from build123d import *

# Parameters (mm, degrees)
F0_W     = 120
F0_H     = 80
F1_DEPTH = 32
F2_W     = 40
F2_H     = 52
F3_DEPTH = 22
F4_W     = 40
F4_H     = 18
F5_DEPTH = 32.001
F6_W     = 30
F6_H     = 70
F7_DEPTH = 32.001
F9_DEPTH = 10


# Not quite as in the source:
# - a pattern or mirror of a feature is missing from the dataset's text; its kind, count and spacing are read off the source's solid


with BuildPart() as f1:
    # F0 (on Right) → F1 (new body)
    with BuildSketch(Plane.YZ):
        Rectangle(F0_W, F0_H)
    extrude(amount=-F1_DEPTH)

    # F2 (on face) → F3 (cut)
    with BuildSketch(Plane.YZ):
        with Locations((0, -14)):
            Rectangle(F2_W, F2_H)
    extrude(amount=-F3_DEPTH, mode=Mode.SUBTRACT)

    # F4 (on face) → F5 (cut, through all)
    with BuildSketch(Plane.YZ):
        with Locations((0, 31)):
            Rectangle(F4_W, F4_H)
    extrude(amount=-F5_DEPTH, mode=Mode.SUBTRACT)

    # F6 (on face) → F7 (cut, through all)
    with BuildSketch(Plane.YZ):
        with Locations((-45, 5)):
            Rectangle(F6_W, F6_H)
    f7 = extrude(amount=-F7_DEPTH, mode=Mode.SUBTRACT)

    # F7_copies: F7 across plane
    add(f7.mirror(Plane.ZX), mode=Mode.SUBTRACT)

    # F8 (on face) → F9 (join)
    with BuildSketch(Plane(origin=(-32, 0, 0), x_dir=(0, -1, 0), z_dir=(-1, 0, 0))):
        Polygon((60, -30), (30, 40), (30, -30), align=None)
    f9 = extrude(amount=-F9_DEPTH)

    # F9_copies: F9 across plane
    add(f9.mirror(Plane.ZX))


solid = f1.part
CAD build for the part. Positions are in the model's coordinates, mm. A direction names the side the tool comes from. Coordinates: 2 decimals unless noted, no trailing zeros. Order: outer loops, then holes, each group sorted by start corner. A loop starts at its lowest first (then second) coordinate and runs counter-clockwise, first axis right, second up.
Item 1: Band-saw the part on A-A on z = 25. List the corners of the cut face in (x, y).
Check sheet entries:
outline: (-32, -36.43) - (-22, -36.43) - (-22, -30) - (0, -30) - (0, -20) - (-32, -20) - close; (-32, 20) - (0, 20) - (0, 30) - (-22, 30) - (-22, 36.43) - (-32, 36.43) - close
Item 2: Pin check, flat tips, straight feed: pin 1 Ø9.5 at (x, y) = (-13.5, -5.5) entering from +Z; pin 2 Ø15 at (y, z) = (-41, 8.5) entering from +X; pin 3 Ø11 at (x, z) = (-8.5, -8.5) entering from -Y. Stop position of each tip, or through.
Check sheet entries:
pin 1: stops at z = 22
pin 2: stops at x = -22
pin 3: stops at y = -30
Item 3: Two-plate mould, pull along Y, no slides. Class faces 4 (the face through (-27, -45, 5)), 5 (the face through (-11, 0, 12)), 6 (the face through (-22, -38, -10)): +Y half, -Y half, draft (parallel to the pull), parting line (faces both ways), or undercut.
Check sheet entries:
face 4: -Y half
face 5: undercut
face 6: draft
Item 4: Band-saw the part on B-B on x = -14.5. List the corners of the cut face in (y, z), plus the area to 3 significant figures.
Check sheet entries:
outline: (-60, -40) - (-20, -40) - (-20, 12) - (20, 12) - (20, -40) - (60, -40) - (60, -30) - (30, -30) - (30, 40) - (20, 40) - (20, 22) - (-20, 22) - (-20, 40) - (-30, 40) - (-30, -30) - (-60, -30) - close
area: 2,600 mm2
Item 5: Band-saw the part on D-D on z = -22.5. List the corners of the cut face in (x, y), plus the area to 3 significant figures.
Check sheet entries:
outline: (-32, -56.79) - (-22, -56.79) - (-22, -30) - (0, -30) - (0, -20) - (-22, -20) - (-22, 20) - (0, 20) - (0, 30) - (-22, 30) - (-22, 56.79) - (-32, 56.79) - close
area: 1,580 mm2
Item 6: Band-saw the part on C-C on y = -48. List the corners of the cut face in (x, z), plus the area to 3 significant figures.
Check sheet entries:
outline: (-32, -40) - (0, -40) - (0, -30) - (-22, -30) - (-22, -2) - (-32, -2) - close
area: 600 mm2
Item 7: 3-axis set-ups, long thin cutter, end or side, ignore diameter. For faces 1 (the face through (-11, -20, -14)), 2 (the face through (-11, -30, 5)), 3 (the face through (-16, 20, 31)): which of +Z, -Z, +X, -X, +Y, -Y reach the whole face in a straight line?
Check sheet entries:
face 1: -Z, +X
face 2: +Z, +X, -Y
face 3: +Z, +X, -X
Item 8: Drill centre lines: L1, parallel to Y at x = -6, z = 23.5; L2, parallel to Y at x = -18, z = -32; L3, parallel to X at y = -38.5, z = -26. Where is each one in solid material? Low to high.
Check sheet entries:
L1: y = -30 to -20, 20 to 30
L2: y = -60 to -20, 20 to 60
L3: x = -32 to -22
